Read the model definition and answer for the solid it produces. Units are mm, in the model's axes. Face numbers are marked on the shaded views. A direction names the side the tool comes from. Coordinates: 2 decimals unless noted, no trailing zeros. Write each loop counter-clockwise with the first axis right and the second up, starting at its lowest first coordinate (ties: lowest second). Pieces come first, ordered by that corner, then holes. Notation, with made-up numbers: (70, 77) -> (96, 77) arc R20 cw to (96, 88) -> close; hole circle Ø5 at (32.25, 31). An arc over 180 degrees is marked (long way). Answer in a Markdown table with one row per item. Add a question column.
Item 1: For a pull along X with two mould halves and no side action, classify the marked faces 3, 4 and 5 as +X half, -X half, draft (parallel to the pull), parting line (faces both ways), or undercut.
Item 2: Section B-B on y = 19 is taken. Write down the section's boundary in (x, z).
Item 3: Section A-A on y = 29 is taken. Write down the section's boundary in (x, z).
Item 4: Which of the six approach directions +Z, -Z, +X, -X, +Y, -Y give full straight-line access (tool end or side, diameter ignored) to the marked faces 1 and 2?
Item 5: Straight lines are drawn through the part: line 1 (Y direction, x = 12, z = 1.25); line 2 (X direction, y = 5.4, z = 0); line 3 (X direction, y = 4.05, z = 0). For each, find the intervals that lie inside material, in ascending order. Write a range as from..to.
Item 6: Given pin 1 Ø4 at (x, y) = (2.5, 23) entering from +Z; pin 2 Ø9.5 at (x, z) = (0, 0) entering from +Y; pin 3 Ø8 at (y, z) = (16.5, -6) entering from +X, each flat-ended and moving along its own axis, determine where each tip first touches the part or whether it passes through.
```python
from build123d import *

# Parameters (mm, degrees)
ESQUISSE4_R             = 3
ENL_V_MAT_EXTRU_3_DEPTH = 43.347845282
CHANFREIN4_SIZE         = 1
CHANFREIN3_SIZE         = 0.5


with BuildPart() as part:
    # Esquisse1 → Révolution1 (revolve)
    with BuildSketch(Plane.XY, mode=Mode.PRIVATE) as r_volution1_sk:
        Polygon((0, 0), (-13.5, 0), (-13.5, 4.64), (-10.73, 4.64), (-10.73, 9.34), (-13.5, 9.34), (-13.5, 16.14), (-10.73, 16.14), (-10.73, 20.84), (-13.5, 20.84), (-13.5, 25.2), (-12.5, 25.2), (-9.5, 25.2), (-9.5, 28.2), (-12.5, 28.2), (-12.5, 31.5), (-9.5, 31.5), (-9.5, 34.5), (-12.5, 34.5), (-12.5, 37.8), (-8, 37.8), (-8, 20.84), (-8, 8), (0, 8), align=None)
    revolve(r_volution1_sk.sketch.rotate(Axis((0, -29.115408637, 0), (0, 1, 0)), 270), axis=Axis((0, -29.115408637, 0), (0, 1, 0)))

    # Esquisse4 → Enlèv. mat.-Extru.3 (cut, through all)
    with BuildSketch(Plane.XZ):
        with Locations(Location((0, 0, 0), (0, 0, 270))):
            Circle(ESQUISSE4_R)
    extrude(amount=-ENL_V_MAT_EXTRU_3_DEPTH, mode=Mode.SUBTRACT)

    # Chanfrein4
    chanfrein4_edges = [part.edges().sort_by_distance(p)[0] for p in [
        (0, 8, 3),
        (0, 0, 3),
    ]]
    chamfer(chanfrein4_edges, length=CHANFREIN4_SIZE)

    # Chanfrein3
    chanfrein3_edges = [part.edges().sort_by_distance(p)[0] for p in [
        (0, 0, 13.5),
        (0, 4.64, 13.5),
        (0, 9.34, 13.5),
        (0, 16.14, 13.5),
        (0, 20.84, 13.5),
    ]]
    chamfer(chanfrein3_edges, length=CHANFREIN3_SIZE)


solid = part.part
```
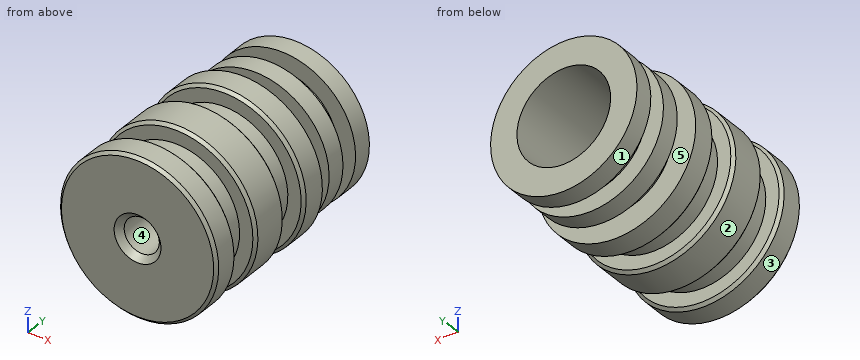
Results below:
| question | item | result |
|---|---|---|
| 1 | face 3 | parting line |
| 1 | face 4 | undercut |
| 1 | face 5 | draft |
| 2 | outline | circle Ø21.46 at (0, 0); hole circle Ø16 at (0, 0) |
| 3 | outline | circle Ø25 at (0, 0); hole circle Ø16 at (0, 0) |
| 4 | face 1 | +Y |
| 4 | face 2 | +Y, -Y |
| 5 | line 1 | y = 0..4.64, 9.34..16.14, 20.84..25.2, 28.2..31.5, 34.5..37.8 |
| 5 | line 2 | x = -10.73..-3, 3..10.73 |
| 5 | line 3 | x = -13.5..-3, 3..13.5 |
| 6 | pin 1 | stops at z = 13.49 |
| 6 | pin 2 | stops at y = 8 |
| 6 | pin 3 | stops at x = 13.34 |
